```python
from build123d import *

# Parameters (mm, degrees)
SKETCH1_W            = 62
SKETCH1_H            = 20
SKETCH1_W_2          = 51.4
SKETCH1_H_2          = 10.4
BOSS_EXTRUDE2_DEPTH  = 3.02
SKETCH3_W            = 62
SKETCH3_H            = 20
BOSS_EXTRUDE3_DEPTH  = 2
SKETCH5_W            = 8.5
SKETCH5_H            = 10.4
CUT_EXTRUDE1_DEPTH   = 10
SKETCH19_W           = 34.4
SKETCH19_H           = 2.300107623
SKETCH19_H_2         = 2.300107622
CUT_EXTRUDE7_DEPTH   = 4
SKETCH21_W           = 7
SKETCH21_H           = 7.100107623
SKETCH21_H_2         = 5.799784755
SKETCH21_H_3         = 7.100107622
SKETCH21_W_2         = 4
BOSS_EXTRUDE11_DEPTH = 2
SKETCH22_R           = 1.5
BOSS_EXTRUDE12_DEPTH = 2.5
FILLET1_R            = 2
FILLET2_R            = 2
SKETCH25_W           = 57.10557297
SKETCH25_H           = 5.799784755
SKETCH25_W_2         = 34.4
BOSS_EXTRUDE13_DEPTH = 3.8
SKETCH26_W           = 57.10557297
SKETCH26_H           = 5.799784755
CUT_EXTRUDE8_DEPTH   = 3.8
SKETCH27_W           = 34.4
SKETCH27_H           = 3.8
CUT_EXTRUDE9_DEPTH   = 20
SKETCH28_W           = 6.2
SKETCH28_H           = 5.799784755
CUT_EXTRUDE10_DEPTH  = 20


with BuildPart() as part:
    # Sketch1 → Boss-Extrude2 (new body)
    with BuildSketch(Plane.XY):
        with Locations((22.463748762, 43.895041876)):
            Rectangle(SKETCH1_W, SKETCH1_H)
        with Locations((22.463748762, 43.895041876)):
            Rectangle(SKETCH1_W_2, SKETCH1_H_2, mode=Mode.SUBTRACT)
    extrude(amount=BOSS_EXTRUDE2_DEPTH)

    # Sketch3 → Boss-Extrude3 (add)
    with BuildSketch(Plane.XY.offset(3.02)):
        with Locations((22.463748762, 43.895041876)):
            Rectangle(SKETCH3_W, SKETCH3_H)
    extrude(amount=BOSS_EXTRUDE3_DEPTH)

    # Sketch5 → Cut-Extrude1 (cut)
    with BuildSketch(Plane(origin=(0, 0, 3.02), x_dir=(-1, 0, 0), z_dir=(0, 0, -1))):
        with Locations((-1.013748762, 43.895041876)):
            Rectangle(SKETCH5_W, SKETCH5_H)
        with Locations((-43.913748762, 43.895041876)):
            Rectangle(SKETCH5_W, SKETCH5_H)
    extrude(amount=-CUT_EXTRUDE1_DEPTH, mode=Mode.SUBTRACT)

    # Sketch19 → Cut-Extrude7 (cut)
    with BuildSketch(Plane.XY.offset(5.02)):
        with Locations((22.463748762, 47.944988065)):
            Rectangle(SKETCH19_W, SKETCH19_H)
        with Locations((22.463748762, 39.845095687)):
            Rectangle(SKETCH19_W, SKETCH19_H_2)
    extrude(amount=-CUT_EXTRUDE7_DEPTH, mode=Mode.SUBTRACT)


with BuildPart() as cut_extrude7_piece_1:
    # of the separate pieces the step leaves, piece 1, a body of its own (cut_extrude7_pieces)
    add(part.part.solids().sort_by_distance((-8.536251238, 33.895041876, 0))[0])



with BuildPart() as cut_extrude7_piece_2:
    # of the separate pieces the step leaves, piece 2, a body of its own (cut_extrude7_pieces)
    add(part.part.solids().sort_by_distance((5.263748762, 46.794934253, 5.02))[0])


with BuildPart() as cut_extrude7_piece_1_1:
    add(cut_extrude7_piece_1.part)

    add(cut_extrude7_piece_2.part)  # Boss-Extrude11 merges Cut-Extrude7 piece 2
    # Sketch21 → Boss-Extrude11 (add)
    with BuildSketch(Plane.XY.offset(5.02)):
        with Locations((29.963748762, 50.344988065)):
            Rectangle(SKETCH21_W, SKETCH21_H)
        with Locations((29.963748762, 43.895041875)):
            Rectangle(SKETCH21_W, SKETCH21_H_2)
        with Locations((29.963748762, 37.445095687)):
            Rectangle(SKETCH21_W, SKETCH21_H_3)
        with Locations((14.963748762, 37.445095687)):
            Rectangle(SKETCH21_W, SKETCH21_H_3)
        with Locations((14.963748762, 43.895041875)):
            Rectangle(SKETCH21_W, SKETCH21_H_2)
        with Locations((14.963748762, 50.344988065)):
            Rectangle(SKETCH21_W, SKETCH21_H)
        with Locations((24.463748762, 50.344988065)):
            Rectangle(SKETCH21_W_2, SKETCH21_H)
        with Locations((24.463748762, 43.895041875)):
            Rectangle(SKETCH21_W_2, SKETCH21_H_2)
        with Locations((24.463748762, 37.445095687)):
            Rectangle(SKETCH21_W_2, SKETCH21_H_3)
        with Locations((20.463748762, 37.445095687)):
            Rectangle(SKETCH21_W_2, SKETCH21_H_3)
        with Locations((20.463748762, 43.895041875)):
            Rectangle(SKETCH21_W_2, SKETCH21_H_2)
        with Locations((20.463748762, 50.344988065)):
            Rectangle(SKETCH21_W_2, SKETCH21_H)
    extrude(amount=-BOSS_EXTRUDE11_DEPTH)

    # Sketch22 → Boss-Extrude12 (add)
    # profile 1 of 2: a face of its own
    with BuildSketch(Plane.XY.offset(5.02)):
        with BuildLine():
            ThreePointArc((53.463748762, 33.895041876), (63.463748762, 43.895041876), (53.463748762, 53.895041876))
            Line((53.463748762, 53.895041876), (53.463748762, 33.895041876))
        make_face()
        with Locations((58.463748762, 43.895041876)):
            Circle(SKETCH22_R, mode=Mode.SUBTRACT)
    # profile 2 of 2: a face of its own
    with BuildSketch(Plane.XY.offset(5.02)):
        with BuildLine():
            ThreePointArc((-8.536251238, 33.895041876), (-18.536251238, 43.895041876), (-8.536251238, 53.895041876))
            Line((-8.536251238, 53.895041876), (-8.536251238, 33.895041876))
        make_face()
        with Locations((-13.536251238, 43.895041876)):
            Circle(SKETCH22_R, mode=Mode.SUBTRACT)
    extrude(amount=-BOSS_EXTRUDE12_DEPTH)

    # Fillet1
    fillet1_edges = [cut_extrude7_piece_1_1.edges().sort_by_distance(p)[0] for p in [
        (53.463748762, 43.895041876, 0),
    ]]
    fillet(fillet1_edges, radius=FILLET1_R)

    # Fillet2
    fillet2_edges = [cut_extrude7_piece_1_1.edges().sort_by_distance(p)[0] for p in [
        (-8.536251238, 43.895041876, 0),
    ]]
    fillet(fillet2_edges, radius=FILLET2_R)

    # Sketch25 → Boss-Extrude13 (add)
    with BuildSketch(Plane.XY.offset(5.02)):
        with Locations((20.043435204, 67.888102351)):
            Rectangle(SKETCH25_W, SKETCH25_H)
        with Locations((22.463748762, 43.895041875)):
            Rectangle(SKETCH25_W_2, SKETCH25_H)
    extrude(amount=BOSS_EXTRUDE13_DEPTH)


with BuildPart() as boss_extrude13_piece_1:
    # of the separate pieces the step leaves, piece 1, a body of its own (boss_extrude13_pieces)
    add(cut_extrude7_piece_1_1.part.solids().sort_by_distance((-6.536251238, 33.895041876, 0))[0])

    # Sketch27 → Cut-Extrude9 (cut)
    with BuildSketch(Plane.XZ.offset(-40.995149498)):
        with Locations((22.463748762, 6.92)):
            Rectangle(SKETCH27_W, SKETCH27_H)
    extrude(amount=-CUT_EXTRUDE9_DEPTH, mode=Mode.SUBTRACT)

    # Sketch28 → Cut-Extrude10 (cut)
    with BuildSketch(Plane.XY.offset(5.02)):
        with Locations((36.563748762, 43.895041875)):
            Rectangle(SKETCH28_W, SKETCH28_H)
        with Locations((8.363748762, 43.895041875)):
            Rectangle(SKETCH28_W, SKETCH28_H)
    extrude(amount=-CUT_EXTRUDE10_DEPTH, mode=Mode.SUBTRACT)


with BuildPart() as boss_extrude13_piece_2:
    # of the separate pieces the step leaves, piece 2, a body of its own (boss_extrude13_pieces)
    add(cut_extrude7_piece_1_1.part.solids().sort_by_distance((-8.509351281, 70.787994728, 5.02))[0])

    # Sketch26 → Cut-Extrude8 (cut)
    with BuildSketch(Plane(origin=(0, 0, 5.02), x_dir=(-1, 0, 0), z_dir=(0, 0, -1))):
        with Locations((-20.043435204, 67.888102351)):
            Rectangle(SKETCH26_W, SKETCH26_H)
    extrude(amount=-CUT_EXTRUDE8_DEPTH, mode=Mode.SUBTRACT)


solid = boss_extrude13_piece_1.part
```
For this review, take the finished solid that the model builds, in its own axes (mm). A direction names the side the tool comes from. Give positions to 0.01 mm unless a question says otherwise; leave off trailing zeros. Order: outer loops, then holes, each group sorted by start corner. A loop starts at its lowest first (then second) coordinate and runs counter-clockwise, first axis right, second up.
1) Take a section at D-D (y = 47.5). Give the boundary of the cut face in (x, z), then the cut area to 3 significant figures.
2) The part is to be moulded in two halves that separate along X. For faces 1 (the face through (11.464, 44, 4)), 2 (the face through (56, 44, 2.52)), 3 (the face through (22, 44, 3.02)), 4 (the face through (-7.935, 44.035, 0.57)), say which applies: released by +X, released by -X, zero draft, split by the parting line, or undercut.
3) For faces 5 (the face through (-11, 44, 2.52)), 6 (the face through (23, 38.695, 2)), 7 (the face through (33.464, 44, 4)), list the 3-axis set-ups (+Z, -Z, +X, -X, +Y, -Y) from which the entire face can be reached by the end or side of a thin tool; tool diameter is ignored.
4) Take a section at A-A (x = 35). Give the boundary of the cut face in (y, z), then the cut area to 3 significant figures.
5) Take a section at B-B (x = 15). Give the boundary of the cut face in (y, z).
6) Wall thickness on line 1 (Y direction, x = 7, z = 1.7); line 2 (X direction, y = 53, z = 1.8); line 3 (Z direction, x = 23.5, y = 40.25): over which ranges is each line inside the solid? List them lowest first.
7) Insertion check: pin 1 (2 mm diameter, centred on y = 42, z = 4, fed in from -X); pin 2 (5 mm diameter, centred on x = 60.5, y = 40, fed in from -Z); pin 3 (3 mm diameter, centred on x = 23, y = 44, fed in from -Z); pin 4 (10 mm diameter, centred on x = 31, y = 49, fed in from -Z). Each pin has a flat end and moves straight along its axis. Give the tip position at first contact, or say it passes through.
8) Take a section at C-C (z = 4.1). Give the boundary of the cut face in (x, y), then the cut area to 3 significant figures.
Derived:
1. outline: (-17.86, 2.52) - (-8.54, 2.52) - (-8.54, 2) arc R2 ccw to (-6.54, 0) - (-3.24, 0) - (-3.24, 5.02) - (-17.86, 5.02) - close; (11.46, 3.02) - (33.46, 3.02) - (33.46, 5.02) - (11.46, 5.02) - close; (48.16, 0) - (51.46, 0) arc R2 ccw to (53.46, 2) - (53.46, 2.52) - (62.79, 2.52) - (62.79, 5.02) - (48.16, 5.02) - close
1. area: 142 mm2
2. face 1: undercut
2. face 2: zero draft
2. face 3: undercut
2. face 4: released by -X
3. face 5: -Z, -X, +Y, -Y
3. face 6: -Z
3. face 7: +Z, -Z
4. outline: (33.9, 0) - (38.7, 0) - (38.7, 5.02) - (33.9, 5.02) - close; (49.1, 0) - (53.9, 0) - (53.9, 5.02) - (49.1, 5.02) - close
4. area: 48.2 mm2
5. outline: (33.9, 0) - (38.7, 0) - (38.7, 3.02) - (49.1, 3.02) - (49.1, 0) - (53.9, 0) - (53.9, 5.02) - (33.9, 5.02) - close
6. line 1: y = 33.9 to 38.7, 49.1 to 53.9
6. line 2: x = -8.53 to 53.45
6. line 3: z = 3.02 to 5.02
7. pin 1: stops at x = -18.5
7. pin 2: stops at z = 2.52
7. pin 3: stops at z = 3.02
7. pin 4: stops at z = 0
8. outline: (-8.54, 33.9) - (53.46, 33.9) arc R10 ccw to (53.46, 53.9) - (-8.54, 53.9) arc R10 ccw to start; hole circle Ø3 at (-13.54, 43.9); hole (-3.24, 38.7) - (11.46, 38.7) - (11.46, 49.1) - (-3.24, 49.1) - close; hole (33.46, 38.7) - (48.16, 38.7) - (48.16, 49.1) - (33.46, 49.1) - close; hole circle Ø3 at (58.46, 43.9)
8. area: 1,230 mm2
